Input: part model. Units: mm. Frame: model coordinates. Coordinates: 2 decimals unless noted, no trailing zeros. Order: outer loops, then holes, each group sorted by start corner. A loop starts at its lowest first (then second) coordinate and runs counter-clockwise, first axis right, second up. Notation, with made-up numbers: (54.5, 85.5) -> (111.5, 85.5) arc R31 cw to (111.5, 114.5) -> close; hole circle Ø6 at (78.5, -0.75). An arc over 180 degrees is marked (long way). Write each question's results on one line, items separated by ' | '.
```python
from build123d import *

# Parameters (mm, degrees)
SKETCH1_R               = 5.685
SKETCH1_R_2             = 3.185
BOSS_EXTRUDE1_DEPTH     = 4.46
SKETCH2_R               = 13
BOSS_EXTRUDE2_DEPTH     = 2.5
SKETCH3_R               = 3.185
CUT_EXTRUDE1_DEPTH      = 2.5
CUT_EXTRUDE3_DEPTH      = 19.918023153
CUT_EXTRUDE3_DEPTH_BACK = 19.918023153


with BuildPart() as part:
    # Sketch1 → Boss-Extrude1 (new body)
    with BuildSketch(Plane(origin=(0, 0, 0), x_dir=(1, 0, 0), z_dir=(0, 1, 0))):
        with Locations(Location((0, 0, 0), (0, 0, 270))):
            Circle(SKETCH1_R)
        with Locations(Location((0, 0, 0), (0, 0, 270))):
            Circle(SKETCH1_R_2, mode=Mode.SUBTRACT)
    extrude(amount=BOSS_EXTRUDE1_DEPTH)

    # Sketch2 → Boss-Extrude2 (add)
    with BuildSketch(Plane(origin=(0, 4.46, 0), x_dir=(1, 0, 0), z_dir=(0, 1, 0))):
        with Locations(Location((0, 0, 0), (0, 0, 270))):
            Circle(SKETCH2_R)
    extrude(amount=BOSS_EXTRUDE2_DEPTH)

    # Sketch3 → Cut-Extrude1 (cut)
    with BuildSketch(Plane.XZ.offset(-4.46)):
        with Locations(Location((0, 0, 0), (0, 0, 270))):
            Circle(SKETCH3_R)
    extrude(amount=-CUT_EXTRUDE1_DEPTH, mode=Mode.SUBTRACT)

    # Sketch4 → Cut-Extrude3 (cut, two sides: drawn at the far end of the back side and taken through both)
    with BuildSketch(Plane.XZ.offset(-4.46).offset(-CUT_EXTRUDE3_DEPTH_BACK)):
        Polygon((-81.445599846, -20.299991547), (-12.85716821, -1.92177668), (-5.685, 0), (-12.407156668, 3.881038962), (-73.901862147, 39.385023724), (-214.796857137, 57.193092978), (-222.340594836, -2.491922293), align=None)
    extrude(amount=CUT_EXTRUDE3_DEPTH + CUT_EXTRUDE3_DEPTH_BACK, mode=Mode.SUBTRACT)


solid = part.part
```
(1) Cut plane A-A, the plane x = 0. Return loops of the section in (y, z) (3 decimals), plus the area to 3 significant figures.
Return value:
outline: (0, -5.685) -> (4.46, -5.685) -> (4.46, -13) -> (6.96, -13) -> (6.96, -3.185) -> (0, -3.185) -> close; (0, 3.185) -> (6.96, 3.185) -> (6.96, 13) -> (4.46, 13) -> (4.46, 5.685) -> (0, 5.685) -> close | area: 71.4 mm2
(2) Mould query, pull axis Z, two halves, no side actions, for faces 1 (the face through (6, 4.46, 0)), 2 (the face through (-5.55, 2.2, -1.23)), 3 (the face through (-8.999, 5.727, 1.913)), 4 (the face through (-9.321, 5.727, -0.974)). Classes: +Z half, -Z half, draft (parallel to the pull), parting line (faces both ways), or undercut.
Return value:
face 1: draft | face 2: parting line | face 3: undercut | face 4: undercut
(3) Cut plane D-D, the plane z = -3.75. Return loops of the section in (x, y).
Return value:
outline: (-12.45, 4.46) -> (-4.27, 4.46) -> (-4.27, 0) -> (4.27, 0) -> (4.27, 4.46) -> (12.45, 4.46) -> (12.45, 6.96) -> (-12.45, 6.96) -> close
(4) Pin query (flat end, axial travel): P1, Ø1.5, axis at y = 5, z = -5, coming from the +X side; P2, Ø4, axis at x = 4, y = 6, coming from the +Z side; P3, Ø6, axis at x = 3.5, z = 8.5, coming from the -Y side. Return the tip coordinate at first contact, or that it passes through.
Return value:
P1: x = 12.29 | P2: z = 12.85 | P3: y = 4.46
(5) Cut plane C-C, the plane x = 3.5. Return loops of the section in (y, z), plus the area to 3 significant figures.
Return value:
outline: (0, -4.48) -> (4.46, -4.48) -> (4.46, -12.52) -> (6.96, -12.52) -> (6.96, 12.52) -> (4.46, 12.52) -> (4.46, 4.48) -> (0, 4.48) -> close | area: 103 mm2
(6) Cut plane B-B, the plane y = 6. Return loops of the section in (x, z) (3 decimals).
Return value:
outline: (-12.857, -1.922) arc R13 ccw (long way) to (-12.407, 3.881) -> (-5.685, 0) -> close; hole circle Ø6.37 at (0, 0)
(7) Line query: line 1 along Z through (x, y) = (0, 6) (3 decimals); line 2 along Z through (x, y) = (0, 1.5) (3 decimals). Output: solid intervals per line, ascending. Write a range as from..to.
Return value:
line 1: -13..-3.185, 3.185..13 | line 2: -5.685..-3.185, 3.185..5.685
